Work out the finished part from the listing and answer in its coordinate system (mm). A direction names the side the tool comes from. Give positions to 0.01 mm unless a question says otherwise; leave off trailing zeros. Loops run counter-clockwise (first coordinate to the right, second up) from the corner with the lowest first, then second, coordinate; pieces in that order, holes last. Notation, with made-up numbers: M 82,-36 L 111,-36 A18 cw 111,-9 Z; hole C 32.5,88 d7. An arc over 180 degrees is marked long. Answer in a Markdown table with one row per item. Add a question column.
from build123d import *

# Parameters (mm, degrees)
BOSS_EXTRU_1_DEPTH      = 10
ESQUISSE3_W             = 9
ESQUISSE3_H             = 75.66
BOSS_EXTRU_2_DEPTH      = 7
ENL_V_MAT_EXTRU_1_DEPTH = 13
ESQUISSE5_RX            = 3.5
ESQUISSE5_RY            = 3
ENL_V_MAT_EXTRU_2_DEPTH = 13
ESQUISSE6_R             = 3.2
ENL_V_MAT_EXTRU_3_DEPTH = 13
ESQUISSE7_R             = 3.5
ENL_V_MAT_EXTRU_4_DEPTH = 13


with BuildPart() as part:
    # Esquisse2 → Boss.-Extru.1 (new body)
    with BuildSketch(Plane.XY):
        Polygon((-14.475776368, 301.567147766), (-14.475776368, 373.567147766), (-5.475776368, 373.567147766), (-5.475776368, 301.567147766), (-5.475776368, 224.004578109), (-14.475776368, 224.004578109), align=None)
    extrude(amount=BOSS_EXTRU_1_DEPTH)

    # Esquisse3 → Boss.-Extru.2 (add)
    with BuildSketch(Plane.XY.offset(10)):
        with Locations((-9.975776368, 261.834578109)):
            Rectangle(ESQUISSE3_W, ESQUISSE3_H)
    extrude(amount=BOSS_EXTRU_2_DEPTH)

    # Esquisse4 → Enlèv. mat.-Extru.1 (cut)
    with BuildSketch(Plane(origin=(-5.475776368, 0, 0), x_dir=(0, 0, -1), z_dir=(1, 0, 0))):
        Polygon((-10, 299.664578109), (-14.659103262, 224.004578109), (-17, 224.004578109), (-17, 299.664578109), align=None)
    extrude(amount=-ENL_V_MAT_EXTRU_1_DEPTH, mode=Mode.SUBTRACT)

    # Esquisse5 → Enlèv. mat.-Extru.2 (cut)
    with BuildSketch(Plane.XY.offset(10)):
        with Locations(Location((-9.975776368, 368.567147766), (0, 0, 90))):
            Ellipse(ESQUISSE5_RX, ESQUISSE5_RY)
    extrude(amount=-ENL_V_MAT_EXTRU_2_DEPTH, mode=Mode.SUBTRACT)

    # Esquisse6 → Enlèv. mat.-Extru.3 (cut)
    with BuildSketch(Plane.XY.offset(10)):
        with Locations((-9.975776368, 368.567147766)):
            Circle(ESQUISSE6_R)
    extrude(amount=-ENL_V_MAT_EXTRU_3_DEPTH, mode=Mode.SUBTRACT)

    # Esquisse7 → Enlèv. mat.-Extru.4 (cut)
    with BuildSketch(Plane(origin=(-5.475776368, 0, 0), x_dir=(0, 0, -1), z_dir=(1, 0, 0))):
        with Locations((-5, 301.567147766)):
            Circle(ESQUISSE7_R)
    extrude(amount=-ENL_V_MAT_EXTRU_4_DEPTH, mode=Mode.SUBTRACT)


solid = part.part
(1) Section C-C, the plane z = 12.5 is taken. Determine the outline of the cut face in (x, y), and give its area (3 significant figures).
(2) The mould has two halves that part along Y. Classify faces 3 (the face through (-13.176, 368.6, 5.07)), 4 (the face through (-10, 337, 10)), 5 (the face through (-10, 373.567, 5)), 6 (the face through (-9.913, 305.037, 5.456)): pulls with the +Y half, pulls with the -Y half, needs draft (parallel to the pull), parting line crosses it, or undercut.
(3) Which of the six approach directions +Z, -Z, +X, -X, +Y, -Y give full straight-line access (tool end or side, diameter ignored) to faces 1 (the face through (-6.776, 368.534, 5.07)), 2 (the face through (-10, 300, 0))?
(4) This flat-tipped pin is pushed along its axis until it touches: P1, Ø4.5, axis at x = -11.5, y = 350.5, coming from the +Z side. Where does it stop, or does it pass through?
(5) Section B-B, the plane y = 244 is taken. Determine the outline of the cut face in (x, z).
(6) Section A-A, the plane z = 5 is taken. State how many separate pieces and enclosed holes the cut face has, and give its area (3 significant figures).
(7) Consider line 1 along Y through (x, z) = (-11.5, 5); line 2 along Y through (x, z) = (-9.5, 5); line 3 along Y through (x, z) = (-10, 1.25). Determine where each line is inside the solid, lowest interval first. Write a range as from..to.
Numbers:
| question | item | result |
|---|---|---|
| 1 | outline | M -14.48,224 L -5.48,224 L -5.48,259.07 L -14.48,259.07 Z |
| 1 | area | 316 mm² |
| 2 | face 3 | undercut |
| 2 | face 4 | needs draft |
| 2 | face 5 | pulls with the +Y half |
| 2 | face 6 | undercut |
| 3 | face 1 | +Z, -Z |
| 3 | face 2 | -Z, +X, -X, +Y, -Y |
| 4 | P1 | stops at z = 10 |
| 5 | outline | M -14.48,0 L -5.48,0 L -5.48,13.43 L -14.48,13.43 Z |
| 6 | separate pieces | 2 |
| 6 | enclosed holes | 1 |
| 6 | area | 1,250 mm² |
| 7 | line 1 | y = 224..298.07, 305.07..365.55, 371.58..373.57 |
| 7 | line 2 | y = 224..298.07, 305.07..365.11, 372.02..373.57 |
| 7 | line 3 | y = 224..365.07, 372.07..373.57 |
